Build history of the part. All positions in model axes, mm. Face numbers are marked on the shaded views. A direction names the side the tool comes from. Give positions to 0.01 mm unless a question says otherwise; leave off trailing zeros. Write each loop counter-clockwise with the first axis right and the second up, starting at its lowest first coordinate (ties: lowest second). Pieces come first, ordered by that corner, then holes.
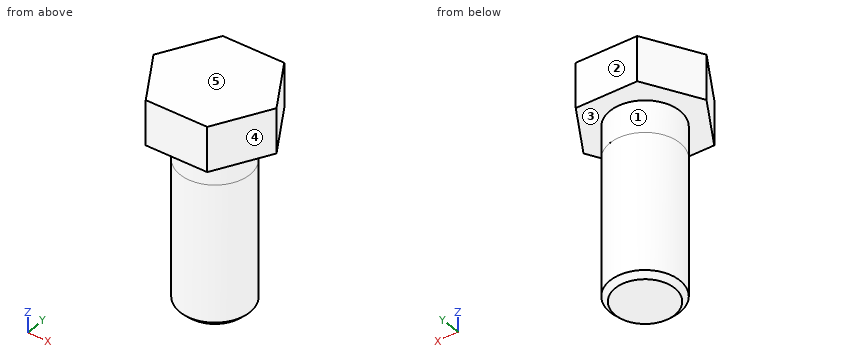
Solid Edge part; units mm, degrees
sketch "Sketch1" plane through (0, 0, 0) normal (0, 0, 1) x (1, 0, 0)
  circle A0 centre (0, 0) radius 10.44
extrude "Protrusion1" add sketch "Sketch1" along normal blind 7.76
sketch "Sketch2" plane through (0, 0, 0) normal (0, 0, -1) x (1, 0, 0)
  circle A0 centre (0, 0) radius 6
extrude "Protrusion2" add sketch "Sketch2" along normal blind 30
sketch "Sketch3" plane through (0, 0, -30) normal (0, 0, -1) x (1, 0, 0)
  circle A0 centre (0, 0) radius 5.9997
extrude "Cutout1" cut sketch "Sketch3" against normal blind 24.5 flip side to cut
chamfer "Chamfer_1" distance 0.9 angle 45 1 edges at (-5.9997, 0, -30)
sketch "Sketch4" plane through (0, 0, 7.76) normal (0, 0, 1) x (1, 0, 0)
  line L0 (-5.2909, 9) -> (5.2909, 9)
extrude "Cutout2" cut sketch "Sketch4" against normal up to next material side at (0, 9.05, 7.76)
pattern_circular "Pattern1" count 6 over 360 about axis through (0, 0, 7.76) along (0, 0, 1) of "Cutout2"
properties part number "118876" material "Stainless Steel, 304"
(1) 3-axis set-ups, long thin cutter, end or side, ignore diameter. For the marked faces 1 and 2: which of +Z, -Z, +X, -X, +Y, -Y reach the whole face in a straight line?
(2) Saw through at D-D, the plane x = 9. List the corners of the cut face in (y, z), plus the area to 3 significant figures.
(3) Mould opens along Z. For the marked faces 3, 4 and 5 say: +Z half, -Z half, draft (parallel to the pull), parting line (faces both ways), or undercut.
(4) Saw through at C-C, the plane z = 4.5. List the corners of the cut face in (x, y).
(5) Probe line 1 (Z direction, x = -4.5, y = 6); line 2 (Y direction, x = 3, z = -21). List the from-to ranges inside material, lowest first.
(6) Drop flat-ended pins along their axis: pin 1 (1.5 mm diameter, centred on y = 6, z = 2.5, fed in from +X); pin 2 (3 mm diameter, centred on y = -7, z = 0, fed in from +X); pin 3 (6 mm diameter, centred on y = 5.5, z = 3, fed in from +X). Give the stop position or say it passes through.
(7) Saw through at B-B, the plane z = -8.5. List the corners of the cut face in (x, y).
Computed values:
1. face 1: -Z
1. face 2: +Z, -Z, +X, -X, +Y
2. outline: (-2.41, 0) - (2.41, 0) - (2.41, 7.76) - (-2.41, 7.76) - close
2. area: 37.4 mm2
3. face 3: -Z half
3. face 4: draft
3. face 5: +Z half
4. outline: (-10.39, 0) - (-5.2, -9) - (5.2, -9) - (10.39, 0) - (5.2, 9) - (-5.2, 9) - close
5. line 1: z = 0 to 7.76
5. line 2: y = -5.2 to 5.2
6. pin 1: stops at x = 7.36
6. pin 2: stops at x = 7.22
6. pin 3: stops at x = 8.95
7. outline: circle Ø12 at (0, 0)
